```python
from build123d import *

# Parameters (mm, degrees)
ESBO_O1_W                = 75
ESBO_O1_H                = 75
RESSALTO_EXTRUS_O1_DEPTH = 1
ESBO_O2_W                = 71
ESBO_O2_H                = 71
ESBO_O2_W_2              = 67
ESBO_O2_H_2              = 67
RESSALTO_EXTRUS_O2_DEPTH = 2
ESBO_O3_W                = 28.5
ESBO_O3_H                = 28.5
ESBO_O3_W_2              = 63
CORTE_EXTRUS_O2_DEPTH    = 3
RESSALTO_EXTRUS_O3_DEPTH = 2


with BuildPart() as part:
    # Esboço1 → Ressalto-extrusão1 (new body)
    with BuildSketch(Plane.XY):
        Rectangle(ESBO_O1_W, ESBO_O1_H)
    extrude(amount=RESSALTO_EXTRUS_O1_DEPTH)

    # Esboço2 → Ressalto-extrusão2 (add)
    with BuildSketch(Plane.XY.offset(1)):
        Rectangle(ESBO_O2_W, ESBO_O2_H)
        Rectangle(ESBO_O2_W_2, ESBO_O2_H_2, mode=Mode.SUBTRACT)
    extrude(amount=RESSALTO_EXTRUS_O2_DEPTH)

    # Esboço3 → Corte-extrusão2 (cut)
    with BuildSketch(Plane.XY.offset(1)):
        with Locations((17.25, 17.25)):
            Rectangle(ESBO_O3_W, ESBO_O3_H)
        with Locations((0, -17.25)):
            Rectangle(ESBO_O3_W_2, ESBO_O3_H)
        with Locations((-17.25, 17.25)):
            Rectangle(ESBO_O3_W, ESBO_O3_H)
    extrude(amount=-CORTE_EXTRUS_O2_DEPTH, mode=Mode.SUBTRACT)

    # Esboço4 → Ressalto-extrusão3 (add)
    with BuildSketch(Plane.XY.offset(1)):
        Polygon((0, 33.5), (-1, 33.5), (-1, 1), (-33.5, 1), (-33.5, 0), (-33.5, -1), (33.5, -1), (33.5, 0), (33.5, 1), (1, 1), (1, 33.5), align=None)
    extrude(amount=RESSALTO_EXTRUS_O3_DEPTH)


solid = part.part
```
Input: part model. Units: mm. Frame: model coordinates. A direction names the side the tool comes from. Round coordinates to 2 decimals unless told otherwise and drop trailing zeros. Write each loop counter-clockwise with the first axis right and the second up, starting at its lowest first coordinate (ties: lowest second). Pieces come first, ordered by that corner, then holes. Notation, with made-up numbers: (-8.5, 27.25) -> (2.5, 27.25) arc R18 cw to (2.5, 49.25) -> close; hole circle Ø9 at (4.25, 66.25). An arc over 180 degrees is marked (long way). Answer as CSV lines item,"result".
1. Contact query for flat-ended pins moving along their axis: P1, Ø1.6, axis at y = -23.5, z = 2, coming from the +X side; P2, Ø0.6, axis at y = 15, z = 2, coming from the -X side; P3, Ø0.6, axis at x = 15.5, z = 2, coming from the +Y side. Output: stop coordinate, or through.
Geometry says:
P1,"stops at x = 35.5"
P2,"stops at x = -35.5"
P3,"stops at y = 35.5"
2. Section B-B (z = 1.8). Return the cut outline in (x, y).
Geometry says:
outline,"(-35.5, -35.5) -> (35.5, -35.5) -> (35.5, 35.5) -> (-35.5, 35.5) -> close; hole (-33.5, -33.5) -> (33.5, -33.5) -> (33.5, -1) -> (-33.5, -1) -> close; hole (-33.5, 1) -> (-1, 1) -> (-1, 33.5) -> (-33.5, 33.5) -> close; hole (1, 1) -> (33.5, 1) -> (33.5, 33.5) -> (1, 33.5) -> close"
3. Section A-A (x = -2). Return the cut outline in (y, z), plus the area to 3 significant figures.
Geometry says:
outline,"(-37.5, 0) -> (-31.5, 0) -> (-31.5, 1) -> (-33.5, 1) -> (-33.5, 3) -> (-35.5, 3) -> (-35.5, 1) -> (-37.5, 1) -> close; (-3, 0) -> (37.5, 0) -> (37.5, 1) -> (35.5, 1) -> (35.5, 3) -> (33.5, 3) -> (33.5, 1) -> (1, 1) -> (1, 3) -> (-1, 3) -> (-1, 1) -> (-3, 1) -> close"
area,"58.5 mm^2"
4. Ray query, L1, parallel to X at y = 2, z = 1.55; L2, parallel to Y at x = 30, z = 0.9. Return the intervals inside material, ascending. Write a range as [from, to].
Geometry says:
L1,"x = [-35.5, -33.5], [-1, 1], [33.5, 35.5]"
L2,"y = [-37.5, -31.5], [-3, 3], [31.5, 37.5]"
5. Section C-C (y = -26). Return the cut outline in (x, z), plus the area to 3 significant figures.
Geometry says:
outline,"(-37.5, 0) -> (-31.5, 0) -> (-31.5, 1) -> (-33.5, 1) -> (-33.5, 3) -> (-35.5, 3) -> (-35.5, 1) -> (-37.5, 1) -> close; (31.5, 0) -> (37.5, 0) -> (37.5, 1) -> (35.5, 1) -> (35.5, 3) -> (33.5, 3) -> (33.5, 1) -> (31.5, 1) -> close"
area,"20.0 mm^2"
6. Mould query, pull axis X, two halves, no side actions, for faces 4 (the flat face through (-33.5, 17, 2)), 5 (the flat face through (35.5, 0, 2)), 6 (the flat face through (0, -35.5, 2)). Classes: +X half, -X half, draft (parallel to the pull), parting line (faces both ways), or undercut.
Geometry says:
face 4,"undercut"
face 5,"+X half"
face 6,"draft"
7. Reachability of faces 1 (the flat face through (1, 17, 2)), 2 (the flat face through (0, 35.5, 2)), 3 (the flat face through (0, 0, 3)) from +Z, -Z, +X, -X, +Y, -Y: full face, straight path, thin tool, end or side. Return the list, or none.
Geometry says:
face 1,"+Z"
face 2,"+Z, +X, -X, +Y"
face 3,"+Z, +X, -X, +Y, -Y"
